from build123d import *

# Parameters (mm, degrees)
SKIZZE1_W   = 2.65
SKIZZE1_H   = 5
SKIZZE2_W   = 1.15
SKIZZE2_H   = 3
FASE1_SIZE  = 0.5
FASE1_SIZE2 = 0.595876796


with BuildPart() as part:
    # Skizze1 → Rotation1 (revolve)
    with BuildSketch(Plane.XY):
        with Locations((-1.325, 0)):
            Rectangle(SKIZZE1_W, SKIZZE1_H)
    revolve(axis=Axis((0, -7.45771041, 0), (0, 1, 0)))

    # Skizze2 → Schnitt-Rotation1 (revolve, cut)
    with BuildSketch(Plane.XY):
        with Locations((-2.075, -1)):
            Rectangle(SKIZZE2_W, SKIZZE2_H)
    revolve(axis=Axis((0, -7.45771041, 0), (0, 1, 0)), mode=Mode.SUBTRACT)

    # Skizze3 → Schnitt-Rotation2 (revolve, cut)
    with BuildSketch(Plane.XY):
        with BuildLine():
            Line((-2.65, 0.5), (-4.39181551, 0.5))
            Line((-4.39181551, 0.5), (-4.39181551, 3.889875423))
            Line((-4.39181551, 3.889875423), (0, 3.889875423))
            Line((0, 3.889875423), (0, 2.5))
            ThreePointArc((0, 2.5), (-1.66000753, 1.943884977), (-2.65, 0.5))
        make_face()
    revolve(axis=Axis((0, -7.45771041, 0), (0, 1, 0)), mode=Mode.SUBTRACT)

    # Fase1
    fase1_edges = [part.edges().sort_by_distance(p)[0] for p in [
        (1.5, -2.5, 0),
    ]]
    fase1_side = [part.faces().sort_by_distance(p)[0] for p in [
        (1.5, -1, 0),
    ]]
    chamfer(fase1_edges, length=FASE1_SIZE, length2=FASE1_SIZE2, reference=fase1_side[0])


solid = part.part
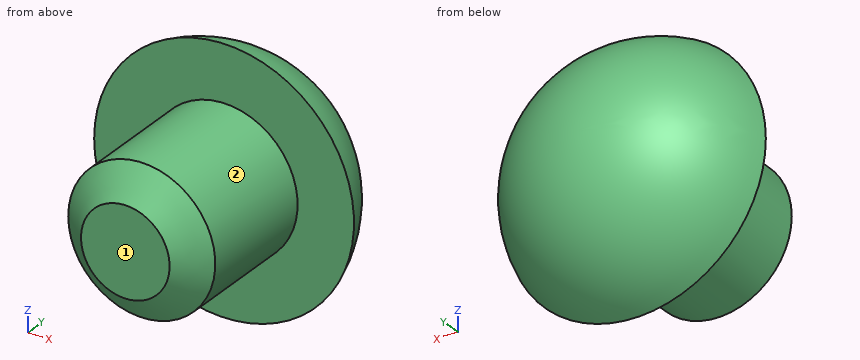
Verification items for the finished model (mm, model axes). Face numbers are marked on the shaded views. A direction names the side the tool comes from. Coordinates: 2 decimals unless noted, no trailing zeros. Order: outer loops, then holes, each group sorted by start corner. A loop starts at its lowest first (then second) coordinate and runs counter-clockwise, first axis right, second up. Notation, with made-up numbers: M -9.75,-3.75 L 39.25,-3.75 A20 ccw 39.25,7.25 Z; hole C 9,48 d8. An arc over 180 degrees is marked long. One line per item, written item: value. Start each with the question number.
Item 1: Sectioned sample at A-A (z = 0). Enter the section's corners in (x, y), then the cut area to 3 significant figures.
Item 2: Gauge pin test, flat ends, axial feed: pin 1 (1.5 mm diameter, centred on x = -2, z = -1.5, fed in from -Y); pin 2 (1.6 mm diameter, centred on x = -1, z = -1, fed in from -Y); pin 3 (2 mm diameter, centred on y = -2, z = -0.5, fed in from +X). Record the tip position at first contact, or that the pin passes through.
Item 3: Scan lines: probe 1 along X at (y, z) = (1.2, 1.05); probe 2 along Z at (x, y) = (-1.15, 1.4); probe 3 along X at (y, z) = (0.6, -0.1). Record each from-to range of solid material in increasing order.
Item 4: Access from +Z, -Z, +X, -X, +Y, -Y to the whole of each face (thin tool, end or side, straight path). Record for the marked faces 1 and 2.
Item 5: Sectioned sample at C-C (y = -1.65). Enter the section's corners in (x, z).
Item 6: Sectioned sample at D-D (x = 1.65). Enter the section's corners in (y, z), then the cut area to 3 significant figures.
Item 7: Sectioned sample at B-B (x = 0). Enter the section's corners in (y, z).
Conclusion:
1. outline: M -2.65,0.5 L -1.5,0.5 L -1.5,-2 L -0.9,-2.5 L 0.9,-2.5 L 1.5,-2 L 1.5,0.5 L 2.65,0.5 A2.76 ccw Z
1. area: 16.5 mm^2
2. pin 1: stops at y = 0.5
2. pin 2: stops at y = -2.5
2. pin 3: stops at x = 1.5
3. probe 1: x = -2.09 to 2.09
3. probe 2: z = -1.88 to 1.88
3. probe 3: x = -2.62 to 2.62
4. face 1: +Z, -Z, +X, -X, -Y
4. face 2: -Y
5. outline: C 0,0 d3
6. outline: M 0.5,-2.07 A2.21 ccw 0.5,2.07 Z
6. area: 4.38 mm^2
7. outline: M -2.5,-0.9 L -2,-1.5 L 0.5,-1.5 L 0.5,-2.65 A2.76 ccw 0.5,2.65 L 0.5,1.5 L -2,1.5 L -2.5,0.9 Z
